Verification items for the finished model (mm, model axes). Face numbers are marked on the shaded views. A direction names the side the tool comes from. Give positions to 0.01 mm unless a question says otherwise; leave off trailing zeros. Write each loop counter-clockwise with the first axis right and the second up, starting at its lowest first coordinate (ties: lowest second). Pieces come first, ordered by that corner, then holes.
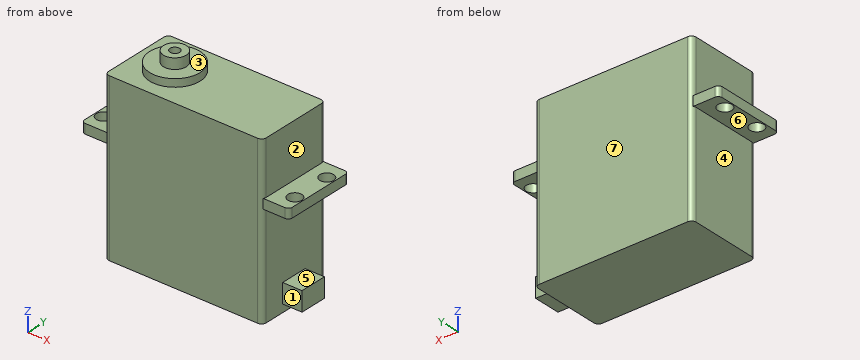
from build123d import *

# Parameters (mm, degrees)
CASE_START   = -42.9
CASE_2_DEPTH = 42.9
TABS_START   = -16.3
SKETCH2_R    = 1.8
TABS_DEPTH   = 2.5
SKETCH3_R    = 6.5
BOSS_DEPTH   = 2
SPLINE_START = 2
SKETCH4_R    = 2.95
SPLINE_DEPTH = 2.7
M3_START     = 0.7
SKETCH5_R    = 1.25
M3_TAP_DEPTH = 4.1
LEAD_START   = 30.5
SKETCH6_W    = 5
SKETCH6_H    = 7
LEAD_DEPTH   = 5.2


with BuildPart() as part:
    # Sketch1 → Case 2 (new body)
    with BuildSketch(Plane.XY.offset(CASE_START)):
        with BuildLine():
            Line((-8.8, -9.85), (29.5, -9.85))
            ThreePointArc((29.5, -9.85), (30.348528137, -9.498528137), (30.7, -8.65))
            Line((30.7, -8.65), (30.7, 8.65))
            ThreePointArc((30.7, 8.65), (30.348528137, 9.498528137), (29.5, 9.85))
            Line((29.5, 9.85), (-8.8, 9.85))
            ThreePointArc((-8.8, 9.85), (-9.648528137, 9.498528137), (-10, 8.65))
            Line((-10, 8.65), (-10, -8.65))
            ThreePointArc((-10, -8.65), (-9.648528137, -9.498528137), (-8.8, -9.85))
        make_face()
    extrude(amount=CASE_2_DEPTH)

    # Sketch2 → Tabs (add)
    with BuildSketch(Plane.XY.offset(TABS_START)):
        with BuildLine():
            Line((-15.45, -9.35), (36.15, -9.35))
            ThreePointArc((36.15, -9.35), (36.857106781, -9.057106781), (37.15, -8.35))
            Line((37.15, -8.35), (37.15, 8.35))
            ThreePointArc((37.15, 8.35), (36.857106781, 9.057106781), (36.15, 9.35))
            Line((36.15, 9.35), (-15.45, 9.35))
            ThreePointArc((-15.45, 9.35), (-16.157106781, 9.057106781), (-16.45, 8.35))
            Line((-16.45, 8.35), (-16.45, -8.35))
            ThreePointArc((-16.45, -8.35), (-16.157106781, -9.057106781), (-15.45, -9.35))
        make_face()
        with Locations((-14.4, -5)):
            Circle(SKETCH2_R, mode=Mode.SUBTRACT)
        with Locations((-14.4, 5)):
            Circle(SKETCH2_R, mode=Mode.SUBTRACT)
        with Locations((35.1, -5)):
            Circle(SKETCH2_R, mode=Mode.SUBTRACT)
        with Locations((35.1, 5)):
            Circle(SKETCH2_R, mode=Mode.SUBTRACT)
    extrude(amount=TABS_DEPTH)

    # Sketch3 → Boss (add)
    with BuildSketch(Plane.XY):
        Circle(SKETCH3_R)
    extrude(amount=BOSS_DEPTH)

    # Sketch4 → Spline (add)
    with BuildSketch(Plane.XY.offset(SPLINE_START)):
        with Locations(Location((0, 0, 0), (0, 0, 180))):
            Circle(SKETCH4_R)
    extrude(amount=SPLINE_DEPTH)

    # Sketch5 → M3 tap (cut)
    with BuildSketch(Plane.XY.offset(M3_START)):
        Circle(SKETCH5_R)
    extrude(amount=M3_TAP_DEPTH, mode=Mode.SUBTRACT)

    # Sketch6 → Lead (add)
    with BuildSketch(Plane(origin=(0, 0, 0), x_dir=(0, 0, -1), z_dir=(1, 0, 0)).offset(LEAD_START)):
        with Locations((38.4, 0)):
            Rectangle(SKETCH6_W, SKETCH6_H)
    extrude(amount=LEAD_DEPTH)


solid = part.part
Item 1: Sectioned sample at C-C on y = -5. Record the cut outline in (x, z), then the cut area to 3 significant figures.
Answer key:
outline: (-16.45, -16.3) - (-16.2, -16.3) - (-16.2, -13.8) - (-16.45, -13.8) - close; (-12.6, -16.3) - (-10, -16.3) - (-10, -42.9) - (30.7, -42.9) - (30.7, -16.3) - (33.3, -16.3) - (33.3, -13.8) - (30.7, -13.8) - (30.7, 0) - (4.15, 0) - (4.15, 2) - (-4.15, 2) - (-4.15, 0) - (-10, 0) - (-10, -13.8) - (-12.6, -13.8) - close; (36.9, -16.3) - (37.15, -16.3) - (37.15, -13.8) - (36.9, -13.8) - close
area: 1,780 mm2
Item 2: Sectioned sample at B-B on z = -15. Record the cut outline in (x, y).
Answer key:
outline: (-16.45, -8.35) arc R1 ccw to (-15.45, -9.35) - (-9.77, -9.35) arc R1.2 ccw to (-8.8, -9.85) - (29.5, -9.85) arc R1.2 ccw to (30.47, -9.35) - (36.15, -9.35) arc R1 ccw to (37.15, -8.35) - (37.15, 8.35) arc R1 ccw to (36.15, 9.35) - (30.47, 9.35) arc R1.2 ccw to (29.5, 9.85) - (-8.8, 9.85) arc R1.2 ccw to (-9.77, 9.35) - (-15.45, 9.35) arc R1 ccw to (-16.45, 8.35) - close; hole circle Ø3.6 at (-14.4, -5); hole circle Ø3.6 at (-14.4, 5); hole circle Ø3.6 at (35.1, -5); hole circle Ø3.6 at (35.1, 5)
Item 3: Release check for a two-part mould opening along Z. For the marked faces 5, 6 and 7 record: released by +Z, released by -Z, zero draft, split by the parting line, or undercut.
Answer key:
face 5: undercut
face 6: released by -Z
face 7: zero draft
Item 4: Sectioned sample at D-D on x = 0. Record the cut outline in (y, z), then the cut area to 3 significant figures.
Answer key:
outline: (-9.85, -42.9) - (9.85, -42.9) - (9.85, 0) - (6.5, 0) - (6.5, 2) - (2.95, 2) - (2.95, 4.7) - (1.25, 4.7) - (1.25, 0.7) - (-1.25, 0.7) - (-1.25, 4.7) - (-2.95, 4.7) - (-2.95, 2) - (-6.5, 2) - (-6.5, 0) - (-9.85, 0) - close
area: 877 mm2
Item 5: Depth check by flat-ended pin: pin 1 (1 mm diameter, centred on x = 30.5, z = -3, fed in from -Y); pin 2 (5.5 mm diameter, centred on x = -12.5, y = -4.5, fed in from +Z); pin 3 (3.5 mm diameter, centred on x = -13.5, y = 2, fed in from -Z); pin 4 (3 mm diameter, centred on x = -14.4, y = 5, fed in from +Z). Enter the tip coordinate at first touch or a pass-through.
Answer key:
pin 1: stops at y = -9.74
pin 2: stops at z = 0
pin 3: stops at z = -16.3
pin 4: passes through
Item 6: Sectioned sample at A-A on x = -14.4. Record the cut outline in (y, z).
Answer key:
outline: (-9.35, -16.3) - (-6.8, -16.3) - (-6.8, -13.8) - (-9.35, -13.8) - close; (-3.2, -16.3) - (3.2, -16.3) - (3.2, -13.8) - (-3.2, -13.8) - close; (6.8, -16.3) - (9.35, -16.3) - (9.35, -13.8) - (6.8, -13.8) - close
Item 7: Set-up check for the marked faces 1, 2, 3 and 4: record each of +Z, -Z, +X, -X, +Y, -Y from which the full face is reachable in a straight line by a thin tool's end or side.
Answer key:
face 1: -Z, +X, -Y
face 2: +Z, +X, +Y, -Y
face 3: +Z
face 4: -Z, -X, +Y, -Y
Item 8: Scan lines: line 1 along Y through (x, z) = (35, -14); line 2 along Z through (x, y) = (18, 2.5). Record each from-to range of solid material in increasing order.
Answer key:
line 1: y = -9.35 to -6.8, -3.2 to 3.2, 6.8 to 9.35
line 2: z = -42.9 to 0
